Geometry: final body of the model. Coordinates: model frame, mm. A direction names the side the tool comes from. Give positions to 0.01 mm unless a question says otherwise; leave off trailing zeros. Write each loop counter-clockwise with the first axis right and the second up, starting at its lowest first coordinate (ties: lowest second). Pieces come first, ordered by that corner, then holes. Notation, with made-up numbers: (62.5, 30.25) -> (92.5, 30.25) arc R24 cw to (92.5, 66.25) -> close; hole circle Ø6 at (88, 4.5). An arc over 180 degrees is marked (long way). Answer as a JSON object with one key per item and string values.
from build123d import *

# Parameters (mm, degrees)
F1_DEPTH = 15
F2_R     = 1.7
F3_DEPTH = 25
F2_R_2   = 2.9
F4_DEPTH = 11


# Not quite as in the source:
# - a feature names something its author has since deleted; it is built from what else it names


with BuildPart() as f1:
    # F0 (on Top) → F1 (new body)
    with BuildSketch(Plane.XY):
        with BuildLine():
            ThreePointArc((3, 2.6457513111), (3.7416573868, 1.4142135624), (4, 0))
            ThreePointArc((4, 0), (-1.4142135624, -3.7416573868), (-3, 2.6457513111))
            ThreePointArc((-3, 2.6457513111), (-2.9417354436, 2.7103860574), (-2.8820786357, 2.7737380442))
            add(Edge.make_bspline(
                [(-2.8820786357, 2.7737380442), (-2.3761359585, 3.4936148761), (-3.7454309361, 4.7943850499), (-4.4301631449, 4.3374709808)],
                knots=[0.118365038, 0.118365038, 0.118365038, 0.118365038, 2.0060809504, 2.0060809504, 2.0060809504, 2.0060809504], degree=3))
            ThreePointArc((-4.4301631449, 4.3374709808), (-4.524697766, 4.2387628061), (-4.6170335889, 4.1379947848))
            ThreePointArc((-4.6170335889, 4.1379947848), (-6.1925482399, 0.3038853354), (-5, -3.666060556))
            ThreePointArc((-5, -3.666060556), (0, -6.2), (5, -3.666060556))
            ThreePointArc((5, -3.666060556), (5.8923679451, -1.9287301522), (6.2, 0))
            ThreePointArc((6.2, 0), (5.7907516028, 2.2152191481), (4.6170335889, 4.1379947848))
            ThreePointArc((4.6170335889, 4.1379947848), (4.524697766, 4.2387628061), (4.4301631449, 4.3374709808))
            add(Edge.make_bspline(
                [(2.8820786357, 2.7737380442), (2.3761359585, 3.4936148761), (3.7454309361, 4.7943850499), (4.4301631449, 4.3374709808)],
                knots=[0.118365038, 0.118365038, 0.118365038, 0.118365038, 2.0060809504, 2.0060809504, 2.0060809504, 2.0060809504], degree=3))
            ThreePointArc((2.8820786357, 2.7737380442), (2.9417354436, 2.7103860574), (3, 2.6457513111))
        make_face()
        with BuildLine():
            ThreePointArc((5, -3.666060556), (0, -6.2), (-5, -3.666060556))
            Line((-5, -3.666060556), (-5, -12.7))
            Line((-5, -12.7), (0, -12.7))
            Line((0, -12.7), (5, -12.7))
            Line((5, -12.7), (5, -3.666060556))
        make_face()
    extrude(amount=F1_DEPTH)

    # F2 (on Front) → F3 (cut)
    with BuildSketch(Plane.XZ):
        with Locations((0, 10.8)):
            Circle(F2_R)
        with Locations((3.5e-09, 4.2)):
            Circle(F2_R)
    extrude(amount=F3_DEPTH, mode=Mode.SUBTRACT)

    # F2 (on Front) → F4 (cut)
    with BuildSketch(Plane.XZ):
        with Locations((0, 10.8)):
            Circle(F2_R_2)
        with Locations((0, 10.8)):
            Circle(F2_R, mode=Mode.SUBTRACT)
        with Locations((3.5e-09, 4.2)):
            Circle(F2_R_2)
        with Locations((3.5e-09, 4.2)):
            Circle(F2_R, mode=Mode.SUBTRACT)
    extrude(amount=F4_DEPTH, mode=Mode.SUBTRACT)


solid = f1.part
Q1. Cut plane C-C (y = -5.5). Return the cut outline in (x, z).
Values:
{"outline": "(-5, 0) -> (5, 0) -> (5, 15) -> (-5, 15) -> close; hole circle Ø5.8 at (0, 4.2); hole circle Ø5.8 at (0, 10.8)"}
Q2. Mould query, pull axis Y, two halves, no side actions, for faces 4 (the cylindrical face through (2.68, -6.82, 9.69)), 5 (the flat face through (-5, -8, 7)), 6 (the flat face through (0, -12.7, 7)). Classes: pulls with the +Y half, pulls with the -Y half, needs draft (parallel to the pull), parting line crosses it, or undercut.
Values:
{"face 4": "undercut", "face 5": "needs draft", "face 6": "pulls with the -Y half"}
Q3. First-contact query: P1, Ø1.7, axis at x = -0.5, z = 12, coming from the +Y side; P2, Ø7, axis at y = -10, z = 11, coming from the +X side; P3, Ø6.5, axis at x = 0, z = 10.8, coming from the +Y side. Flat tips, straight axial feed; report the tip coordinate or a pass-through.
Values:
{"P1": "y = -11", "P2": "x = 5", "P3": "y = 4.04"}
Q4. Material intervals for L1, parallel to Z at x = 0, y = -12; L2, parallel to Z at x = 0, y = -8; L3, parallel to X at y = -12.3, z = 4.2, sorted ascending. Write a range as from..to.
Values:
{"L1": "0..2.5, 5.9..9.1, 12.5..15", "L2": "0..1.3, 7.1..7.9, 13.7..15", "L3": "-5..-1.7, 1.7..5"}
Q5. Set-up query: faces 1 (the cylindrical face through (2.766, -6.82, 5.071)), 2 (the cylindrical face through (0.914, -11.838, 5.633)), 3 (the flat face through (5, -8, 7)). Return all of +Z, -Z, +X, -X, +Y, -Y with unobstructed straight access to the full face (end or side cutting, diameter ignored); none if empty.
Values:
{"face 1": "none", "face 2": "+Y, -Y", "face 3": "+Z, -Z, +X, -Y"}
Q6. Cut plane B-B (y = -0.5). Return the cut outline in (x, z), and give its area (3 significant figures).
Values:
{"outline": "(-6.18, 0) -> (-3.97, 0) -> (-3.97, 15) -> (-6.18, 15) -> close; (3.97, 0) -> (6.18, 0) -> (6.18, 15) -> (3.97, 15) -> close", "area": "66.3 mm²"}
Q7. Cut plane A-A (x = 0). Return the cut outline in (y, z), and give its area (3 significant figures).
Values:
{"outline": "(-12.7, 0) -> (-4, 0) -> (-4, 1.3) -> (-11, 1.3) -> (-11, 2.5) -> (-12.7, 2.5) -> close; (-12.7, 5.9) -> (-11, 5.9) -> (-11, 7.1) -> (-4, 7.1) -> (-4, 7.9) -> (-11, 7.9) -> (-11, 9.1) -> (-12.7, 9.1) -> close; (-12.7, 12.5) -> (-11, 12.5) -> (-11, 13.7) -> (-4, 13.7) -> (-4, 15) -> (-12.7, 15) -> close", "area": "37.7 mm²"}
